Input: part model. Units: mm. Frame: model coordinates. A direction names the side the tool comes from. Give positions to 0.01 mm unless a question says otherwise; leave off trailing zeros. Order: outer loops, then holes, each group sorted by start corner. A loop starts at its lowest first (then second) coordinate and runs counter-clockwise, first axis right, second up. Notation, with made-up numbers: (38.25, 35.5) -> (46.25, 35.5) arc R10 ccw to (46.25, 41.5) -> close; hole circle Ø10 at (-8, 79). An arc over 180 degrees is marked (long way). Use a Markdown table: item, result. Add a question column.
from build123d import *

# Parameters (mm, degrees)
SKETCH1_R           = 4
SKETCH1_R_2         = 1.05
BOSS_EXTRUDE1_DEPTH = 4
SKETCH2_R           = 2.5
BOSS_EXTRUDE2_DEPTH = 1
SKETCH1_2_R         = 1.05
CUT_EXTRUDE1_DEPTH  = 8.549834435
FILLET1_R           = 0.5


with BuildPart() as part:
    # Sketch1 → Boss-Extrude1 (new body)
    with BuildSketch(Plane(origin=(0, 0, 0), x_dir=(1, 0, 0), z_dir=(0, 1, 0))):
        with Locations(Location((0, 0, 0), (0, 0, 270))):
            Circle(SKETCH1_R)
        with Locations(Location((0, 0, 0), (0, 0, 270))):
            Circle(SKETCH1_R_2, mode=Mode.SUBTRACT)
    extrude(amount=BOSS_EXTRUDE1_DEPTH)

    # Sketch2 → Boss-Extrude2 (add)
    with BuildSketch(Plane(origin=(0, 4, 0), x_dir=(1, 0, 0), z_dir=(0, 1, 0))):
        with Locations(Location((0, 0, 0), (0, 0, 270))):
            Circle(SKETCH2_R)
    extrude(amount=BOSS_EXTRUDE2_DEPTH)

    # Sketch1_2 → Cut-Extrude1 (cut, through all)
    with BuildSketch(Plane(origin=(0, 0, 0), x_dir=(1, 0, 0), z_dir=(0, 1, 0))):
        with Locations(Location((0, 0, 0), (0, 0, 270))):
            Circle(SKETCH1_2_R)
    extrude(amount=CUT_EXTRUDE1_DEPTH, mode=Mode.SUBTRACT)

    # Fillet1
    fillet1_edges = [part.edges().sort_by_distance(p)[0] for p in [
        (0, 5, -1.05),
        (0, 0, -1.05),
    ]]
    fillet(fillet1_edges, radius=FILLET1_R)


solid = part.part
Q1. Section query C-C (y = 2.05). Return loops of the section in (x, z).
Q2. Section query D-D (x = -2). Return loops of the section in (y, z).
Q3. Draft query along X for faces 3 (the flat face through (0, 0, 2)), 4 (the cylindrical face through (-2.44, 4.49, -0.54)), 5 (the cylindrical face through (0.32, 2.47, 1)). Return one class per face: +X half, -X half, draft (parallel to the pull), parting line (faces both ways), or undercut.
Q4. First-contact query: pin 1 (3 mm diameter, centred on y = 1.5, z = -3, fed in from -X); pin 2 (1.5 mm diameter, centred on y = 4, z = 2.5, fed in from -X); pin 3 (1.5 mm diameter, centred on x = 3, y = 3.5, fed in from -Z). Flat tips, straight axial feed; report the tip coordinate or a pass-through.
Q5. Section query B-B (z = 0). Return loops of the section in (x, y).
Q6. Section query A-A (x = 0). Return loops of the section in (y, z).
Q7. Access query for faces 1 (the cylindrical face through (-3.905, 1.972, -0.867)), 2 (the flat face through (2, 4, 2)). Directions: +Z, -Z, +X, -X, +Y, -Y. A direction counts if a zero-diameter tool reaches every point of the face in a straight line with its end or side. Return the directions, or none.
Q8. Ray query, line 1 (X direction, y = 2.3, z = 0); line 2 (Y direction, x = -2.5, z = -1.75); line 3 (Z direction, x = -0.75, y = 0.3). Return the intervals inside material, ascending.
Solution:
| question | item | result |
|---|---|---|
| 1 | outline | circle Ø8 at (0, 0); hole circle Ø2.1 at (0, 0) |
| 2 | outline | (0, -3.46) -> (4, -3.46) -> (4, -1.5) -> (5, -1.5) -> (5, 1.5) -> (4, 1.5) -> (4, 3.46) -> (0, 3.46) -> close |
| 3 | face 3 | draft |
| 3 | face 4 | parting line |
| 3 | face 5 | undercut |
| 4 | pin 1 | stops at x = -3.71 |
| 4 | pin 2 | stops at x = -3.6 |
| 4 | pin 3 | stops at z = -3.31 |
| 5 | outline | (-4, 0) -> (-1.55, 0) arc R0.5 ccw to (-1.05, 0.5) -> (-1.05, 4.5) arc R0.5 ccw to (-1.55, 5) -> (-2.5, 5) -> (-2.5, 4) -> (-4, 4) -> close; (1.05, 0.5) arc R0.5 ccw to (1.55, 0) -> (4, 0) -> (4, 4) -> (2.5, 4) -> (2.5, 5) -> (1.55, 5) arc R0.5 ccw to (1.05, 4.5) -> close |
| 6 | outline | (0, -4) -> (4, -4) -> (4, -2.5) -> (5, -2.5) -> (5, -1.55) arc R0.5 ccw to (4.5, -1.05) -> (0.5, -1.05) arc R0.5 ccw to (0, -1.55) -> close; (0, 1.55) arc R0.5 ccw to (0.5, 1.05) -> (4.5, 1.05) arc R0.5 ccw to (5, 1.55) -> (5, 2.5) -> (4, 2.5) -> (4, 4) -> (0, 4) -> close |
| 7 | face 1 | +Y, -Y |
| 7 | face 2 | +Y |
| 8 | line 1 | x = -4 to -1.05, 1.05 to 4 |
| 8 | line 2 | y = 0 to 4 |
| 8 | line 3 | z = -3.93 to -0.79, 0.79 to 3.93 |
